from build123d import *

# Parameters (mm, degrees)
F0_W     = 57.635396
F0_H     = 55.43743
F0_W_2   = 45.91294
F0_H_2   = 41.272804
F1_DEPTH = 25
F2_W     = 57.635396
F2_H     = 55.43743
F3_DEPTH = 10
F4_W     = 57.635396
F4_H     = 37.36532
F5_DEPTH = 25


with BuildPart() as f1:
    # F0 (on Top) → F1 (new body)
    with BuildSketch(Plane.XY):
        Rectangle(F0_W, F0_H)
        Rectangle(F0_W_2, F0_H_2, mode=Mode.SUBTRACT)
    extrude(amount=F1_DEPTH)

    # F2 (on face) → F3 (join)
    with BuildSketch(Plane(origin=(0, 0, 0), x_dir=(1, 0, 0), z_dir=(0, 0, -1))):
        Rectangle(F2_W, F2_H)
    extrude(amount=F3_DEPTH)

    # F4 (on face) → F5 (join)
    with BuildSketch(Plane(origin=(0, 0, -10), x_dir=(1, 0, 0), z_dir=(0, 0, -1))):
        with Locations((0, -9.036055)):
            Rectangle(F4_W, F4_H)
    extrude(amount=F5_DEPTH)


solid = f1.part
Input: part model. Units: mm. Frame: model coordinates. A direction names the side the tool comes from. Give positions to 0.01 mm unless a question says otherwise; leave off trailing zeros. Order: outer loops, then holes, each group sorted by start corner. A loop starts at its lowest first (then second) coordinate and runs counter-clockwise, first axis right, second up. Notation, with made-up numbers: (11, 60.25) - (57, 60.25) arc R9 ccw to (57, 66.25) - close; hole circle Ø11 at (-14, 18). An arc over 180 degrees is marked (long way). Write each question's results on one line, items separated by ' | '.
Item 1: Section D-D (z = -30). Return loops of the section in (x, y).
A:
outline: (-28.82, -9.65) - (28.82, -9.65) - (28.82, 27.72) - (-28.82, 27.72) - close
Item 2: Draft query along X for faces 1 (the flat face through (28.818, 7, -5)), 2 (the flat face through (0, -24, 25)), 3 (the flat face through (0, -20.636, 12)). Return one class per face: released by +X, released by -X, zero draft, split by the parting line, or undercut.
A:
face 1: released by +X | face 2: zero draft | face 3: undercut
Item 3: Material intervals for line 1 along X through (y, z) = (0, 22); line 2 along Y through (x, z) = (-19.5, 7.5); line 3 along Z through (x, y) = (-1, -12.5), sorted ascending.
A:
line 1: x = -28.82 to -22.96, 22.96 to 28.82 | line 2: y = -27.72 to -20.64, 20.64 to 27.72 | line 3: z = -10 to 0
Item 4: Section B-B (y = -11). Return loops of the section in (x, z).
A:
outline: (-28.82, -10) - (28.82, -10) - (28.82, 25) - (22.96, 25) - (22.96, 0) - (-22.96, 0) - (-22.96, 25) - (-28.82, 25) - close
Item 5: Section C-C (x = -6.5). Return loops of the section in (y, z), and give its area (3 significant figures).
A:
outline: (-27.72, -10) - (-9.65, -10) - (-9.65, -35) - (27.72, -35) - (27.72, 25) - (20.64, 25) - (20.64, 0) - (-20.64, 0) - (-20.64, 25) - (-27.72, 25) - close | area: 1,840 mm^2
Item 6: Access query for faces 4 (the flat face through (0, -27.719, 8)), 5 (the flat face through (0, -9.647, -22)), 6 (the flat face through (0, 0, 0)). Directions: +Z, -Z, +X, -X, +Y, -Y. A direction counts if a zero-diameter tool reaches every point of the face in a straight line with its end or side. Return the directions, or none.
A:
face 4: +Z, -Z, +X, -X, -Y | face 5: -Z, +X, -X, -Y | face 6: +Z
Item 7: Section A-A (z = 7). Return loops of the section in (x, y), and give its area (3 significant figures).
A:
outline: (-28.82, -27.72) - (28.82, -27.72) - (28.82, 27.72) - (-28.82, 27.72) - close; hole (-22.96, -20.64) - (22.96, -20.64) - (22.96, 20.64) - (-22.96, 20.64) - close | area: 1,300 mm^2
Item 8: Contact query for flat-ended pins moving along their axis: pin 1 Ø3 at (x, y) = (3, -15.5) entering from +Z; pin 2 Ø12 at (x, z) = (-4.5, -22.5) entering from -Y; pin 3 Ø5.5 at (x, y) = (-7.5, -14.5) entering from -Z. Output: stop coordinate, or through.
A:
pin 1: stops at z = 0 | pin 2: stops at y = -9.65 | pin 3: stops at z = -10
